Work out the finished part from the listing and answer in its coordinate system (mm). Face numbers are marked on the shaded views. Coordinates: 2 decimals unless noted, no trailing zeros. Write each loop counter-clockwise with the first axis right and the second up, starting at its lowest first coordinate (ties: lowest second). Pieces come first, ordered by that corner, then holes. Notation, with made-up numbers: (41, -23.5) - (68, -23.5) arc R19 cw to (68, 3.5) - close; hole circle Ø3 at (49.5, 13). An arc over 180 degrees is marked (long way). One line per item, written item: value.
```python
from build123d import *

# Parameters (mm, degrees)
EXTRUDE_1_DEPTH     = 5
SKETCH_2_R          = 4
CUT_EXTRUDE_1_DEPTH = 10


with BuildPart() as part:
    # 草图1 → 凸台-拉伸1 (new body)
    with BuildSketch(Plane.XY):
        Polygon((35, 0), (-35, 0), (-65, 30), (-90, 30), (-90, 50), (-55, 50), (-25, 20), (25, 20), (55, 50), (90, 50), (90, 30), (65, 30), align=None)
    extrude(amount=EXTRUDE_1_DEPTH)

    # 草图2 → 切除-拉伸1 (cut)
    with BuildSketch(Plane(origin=(0, 0, 0), x_dir=(-1, 0, 0), z_dir=(0, 0, -1))):
        with Locations((70, 40)):
            Circle(SKETCH_2_R)
        with Locations(Location((-70, 40, 0), (0, 0, 180))):
            Circle(SKETCH_2_R)
    extrude(amount=-CUT_EXTRUDE_1_DEPTH, mode=Mode.SUBTRACT)


solid = part.part
```
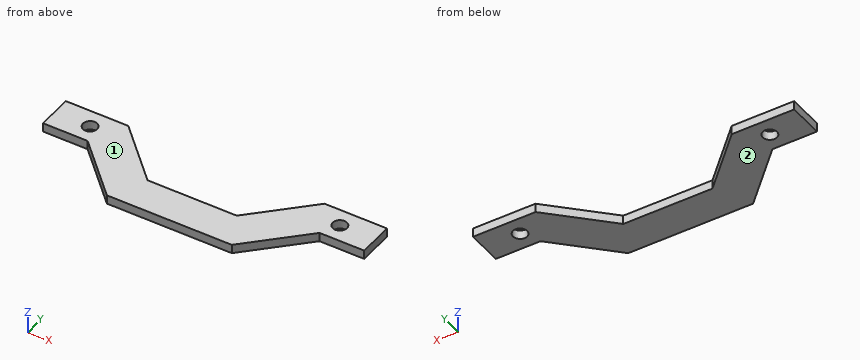
Item 1: Section B-B, the plane x = 70 is taken. Determine the outline of the cut face in (y, z).
Evaluation:
outline: (30, 0) - (36, 0) - (36, 5) - (30, 5) - close; (44, 0) - (50, 0) - (50, 5) - (44, 5) - close
Item 2: Consider probe 1 along Y at (x, z) = (70, 1.95); probe 2 along X at (y, z) = (42, 1.7); probe 3 along X at (y, z) = (27, 2). Determine where each line is inside the solid, lowest interval first.
Evaluation:
probe 1: y = 30 to 36, 44 to 50
probe 2: x = -90 to -73.46, -66.54 to -47, 47 to 66.54, 73.46 to 90
probe 3: x = -62 to -32, 32 to 62
Item 3: Section A-A, the plane y = 40 is taken. Determine the outline of the cut face in (x, z).
Evaluation:
outline: (-90, 0) - (-74, 0) - (-74, 5) - (-90, 5) - close; (-66, 0) - (-45, 0) - (-45, 5) - (-66, 5) - close; (45, 0) - (66, 0) - (66, 5) - (45, 5) - close; (74, 0) - (90, 0) - (90, 5) - (74, 5) - close
Item 4: Given pin 1 (1.5 mm diameter, centred on x = 73, z = 3, fed in from -Y); pin 2 (6.5 mm diameter, centred on x = 70, y = 40, fed in from +Z); pin 3 (2.5 mm diameter, centred on x = 4, z = 2, fed in from +Y); pin 4 (1 mm diameter, centred on x = -38.5, y = 6, fed in from -Z), each flat-ended and moving along its own axis, determine where each tip first touches the part or whether it passes through.
Evaluation:
pin 1: stops at y = 30
pin 2: passes through
pin 3: stops at y = 20
pin 4: stops at z = 0
Item 5: Section C-C, the plane z = 4.25 is taken. Determine the outline of the cut face in (x, y).
Evaluation:
outline: (-90, 30) - (-65, 30) - (-35, 0) - (35, 0) - (65, 30) - (90, 30) - (90, 50) - (55, 50) - (25, 20) - (-25, 20) - (-55, 50) - (-90, 50) - close; hole circle Ø8 at (-70, 40); hole circle Ø8 at (70, 40)
Item 6: Section D-D, the plane x = 39.5 is taken. Determine the outline of the cut face in (y, z), then the cut area to 3 significant figures.
Evaluation:
outline: (4.5, 0) - (34.5, 0) - (34.5, 5) - (4.5, 5) - close
area: 150 mm2
Item 7: Determine the mould class of the marked faces 1 and 2 for opening direction Z: +Z half, -Z half, draft (parallel to the pull), parting line (faces both ways), or undercut.
Evaluation:
face 1: +Z half
face 2: -Z half
